Geometry check sheet. Reference: drawing and pictorial views, mm from the part's lowest x, y, z. A direction names the side the tool comes from. Give positions to 0.01 mm unless a question says otherwise; leave off trailing zeros. Write each question's results on one line, items separated by ' | '. Start each with the question number.
1. Mould release check, pull along X, two halves, no side actions. Record for the marked faces 1, 2 and 3: +X half, -X half, draft (parallel to the pull), parting line (faces both ways), or undercut.
2. Tool access check on the marked faces 4 and 5. Record the directions out of +Z, -Z, +X, -X, +Y, -Y that give a thin tool (end or side, any length) a straight path to the whole face; none if there is none.
3. Gauge pin test, flat ends, axial feed: pin 1 Ø1.5 at (y, z) = (1.5, 26.5) entering from -X; pin 2 Ø1.8 at (x, z) = (18.25, 18.25) entering from -Y. Record the tip position at first contact, or that the pin passes through.
4. Material ranges on L1, parallel to Z at x = 6.5, y = 2.2 (1 decimal); L2, parallel to Y at x = 10.5, z = 13; L3, parallel to Z at x = 22, y = 3.3 (1 decimal), recorded low to high. Write a range as from..to.
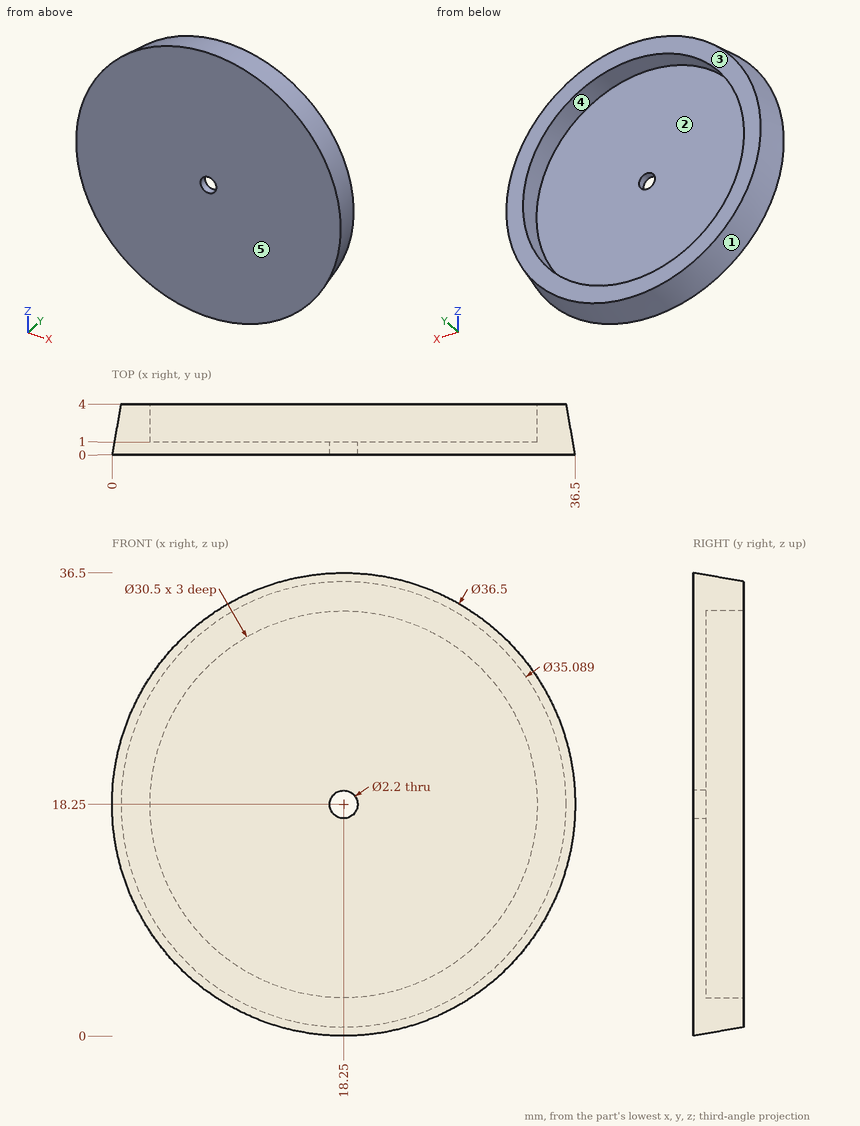
Geometry says:
1) face 1: parting line | face 2: undercut | face 3: draft
2) face 4: +Y | face 5: +Z, -Z, +X, -X, -Y
3) pin 1: x = 1.87 | pin 2: through
4) L1: 4.8..8.5, 28..31.7 | L2: 0..1 | L3: 1..3.5, 33..35.5
